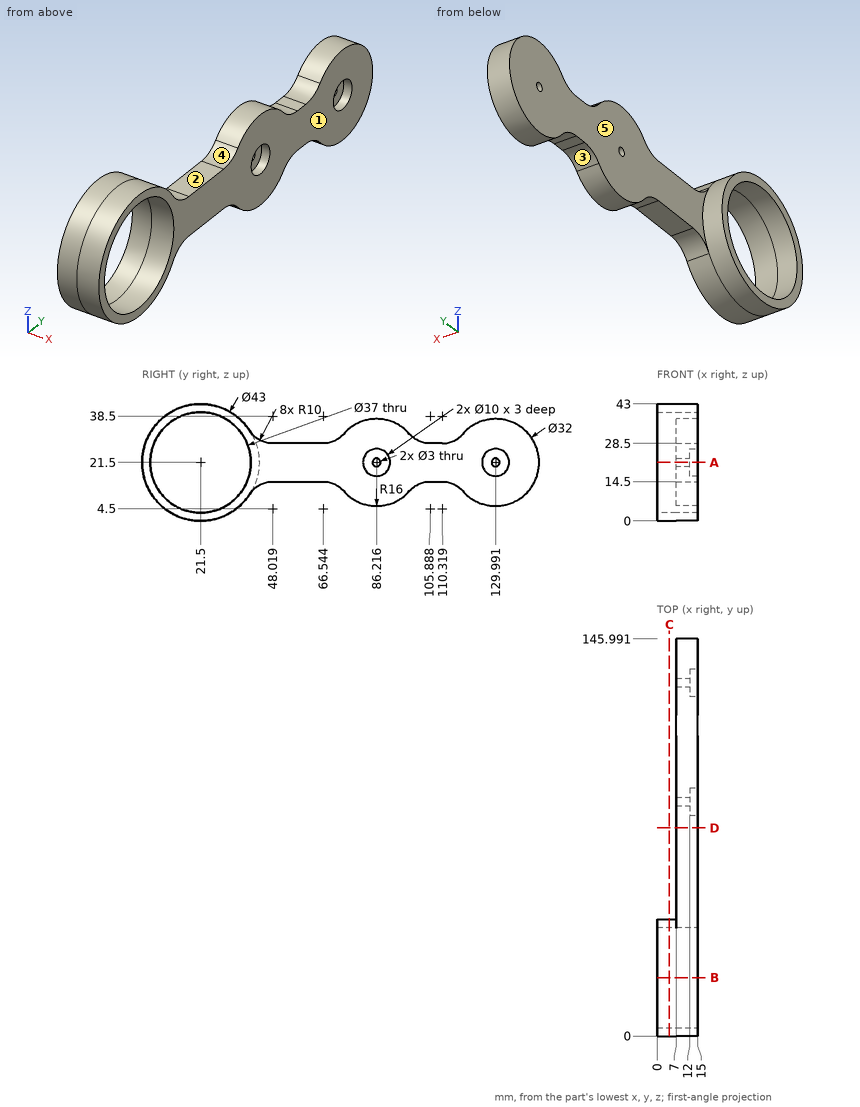
Check sheet for the drawn part. Datum: minimum x, y, z corner. Units: mm. A direction names the side the tool comes from. Round coordinates to 2 decimals unless told otherwise and drop trailing zeros. Order: outer loops, then holes, each group sorted by start corner. A loop starts at its lowest first (then second) coordinate and runs counter-clockwise, first axis right, second up. Notation, with made-up numbers: (88, 62) -> (94, 62) arc R18 cw to (94, 67) -> close; hole circle Ø1 at (88, 72). An arc over 180 degrees is marked (long way). Put each result on its own line as item: value.
1) Section check D-D (y = 76.5). Record the cut outline in (x, z).
Final values:
outline: (7, 8.79) -> (15, 8.79) -> (15, 34.21) -> (7, 34.21) -> close
2) Section check B-B (y = 21.5). Record the cut outline in (x, z).
Final values:
outline: (0, 0) -> (15, 0) -> (15, 3) -> (0, 3) -> close; (0, 40) -> (15, 40) -> (15, 43) -> (0, 43) -> close
3) Section check A-A (z = 21.5). Record the cut outline in (x, y), then the cut area to 3 significant figures.
Final values:
outline: (0, 0) -> (15, 0) -> (15, 3) -> (0, 3) -> close; (0, 40) -> (15, 40) -> (15, 81.22) -> (12, 81.22) -> (12, 84.72) -> (7, 84.72) -> (7, 43) -> (0, 43) -> close; (7, 87.72) -> (12, 87.72) -> (12, 91.22) -> (15, 91.22) -> (15, 124.99) -> (12, 124.99) -> (12, 128.49) -> (7, 128.49) -> close; (7, 131.49) -> (12, 131.49) -> (12, 134.99) -> (15, 134.99) -> (15, 145.99) -> (7, 145.99) -> close
area: 824 mm^2
4) Mould release check, pull along Y, two halves, no side actions. Record for the marked faces 4 and 5: +Y half, -Y half, draft (parallel to the pull), parting line (faces both ways), or undercut.
Final values:
face 4: undercut
face 5: draft
5) Set-up check for the marked faces 1, 2 and 3: record each of +Z, -Z, +X, -X, +Y, -Y from which the full face is reachable in a straight line by a thin tool's end or side.
Final values:
face 1: +Z, -Z, +X, +Y, -Y
face 2: +Z, +X, -X
face 3: -Z, +X, -X
6) Depth check by flat-ended pin: pin 1 (4 mm diameter, centred on x = 6.5, z = 27, fed in from +Y); pin 2 (6 mm diameter, centred on y = 86.22, z = 21.5, fed in from +X); pin 3 (3.5 mm diameter, centred on x = 12.5, y = 107.5, fed in from +Z). Enter the tip coordinate at first touch or a pass-through.
Final values:
pin 1: stops at y = 145.59
pin 2: stops at x = 12
pin 3: stops at z = 28.5
7) Material ranges on line 1 (Y direction, x = 9.5, z = 21.5); line 2 (Y direction, x = 13.4, z = 21.5); line 3 (Y direction, x = 5.25, z = 21.5), recorded low to high.
Final values:
line 1: y = 0 to 3, 40 to 84.72, 87.72 to 128.49, 131.49 to 145.99
line 2: y = 0 to 3, 40 to 81.22, 91.22 to 124.99, 134.99 to 145.99
line 3: y = 0 to 3, 40 to 43
8) Section check C-C (x = 4.5). Record the cut outline in (y, z).
Final values:
outline: circle Ø43 at (21.5, 21.5); hole circle Ø37 at (21.5, 21.5)
